from build123d import *

# Parameters (mm, degrees)
F2_W     = 2.54
F2_H     = 5.588
F3_DEPTH = 9.525
F5_D     = 3.2
F5_DEPTH = 7.5067


with BuildPart() as f1:
    # F0 (on Front) → F1 (revolve)
    with BuildSketch(Plane.XZ):
        Polygon((2.6, 17), (2.6, 0), (7.5057, 0), (7.5057, 15), (6.25, 15), (6.25, 17), align=None)
    revolve(axis=Axis((0, 0, 12.7238426358), (0, 0, -1)))

    # F2 (on face) → F3 (cut)
    with BuildSketch(Plane(origin=(0, 0, 0), x_dir=(1, 0, 0), z_dir=(0, 0, -1))):
        with Locations((5.08, 0)):
            Rectangle(F2_W, F2_H)
    extrude(amount=-F3_DEPTH, mode=Mode.SUBTRACT)

    # F5 (through all, one way)
    with BuildSketch(Plane(origin=(0, 0, 0), x_dir=(0, 1, 0), z_dir=(-1, 0, 0))):
        with Locations((0, -4.7625)):
            Circle(F5_D / 2)
    extrude(amount=-F5_DEPTH, mode=Mode.SUBTRACT)


solid = f1.part
CAD build for the part. Positions are in the model's coordinates, mm. A direction names the side the tool comes from. Round coordinates to 2 decimals unless told otherwise and drop trailing zeros. Write each loop counter-clockwise with the first axis right and the second up, starting at its lowest first coordinate (ties: lowest second). Pieces come first, ordered by that corner, then holes. Notation, with made-up numbers: (-4, 55.25) -> (43, 55.25) arc R22 ccw to (43, 67.25) -> close; hole circle Ø3 at (23.5, 21). An arc over 180 degrees is marked (long way). Answer as a JSON object with one key per item and string values.
(1) Pin check, flat tips, straight feed: P1, Ø3, axis at x = 5, z = 3.5, coming from the +Y side; P2, Ø3, axis at x = 5.5, z = 4.5, coming from the -Y side; P3, Ø1.5, axis at y = 3, z = 4.5, coming from the -X side. Stop position of each tip, or through.
Reported:
{"P1": "stops at y = 6.64", "P2": "stops at y = -6.35", "P3": "stops at x = -7.16"}
(2) Which spindle directions (+Z, -Z, +X, -X, +Y, -Y) get a long thin tool onto all of the face, cutting with end or side? Do faces 4 (the face through (-3, -6, 15)), 5 (the face through (6.35, 2, 5)), 6 (the face through (0, 3, 17)), 7 (the face through (-2.6, -0.1, 8.4)), 8 (the face through (3.11, -1.18, 3.68)). Say none if no direction does.
Reported:
{"face 4": "+Z", "face 5": "-Z", "face 6": "+Z, +X, -X, +Y, -Y", "face 7": "+Z, -Z", "face 8": "+X"}
(3) Band-saw the part on C-C, the plane y = -2.25. List the corners of the cut face in (x, z) (3 decimals).
Reported:
{"outline": "(-7.161, 0) -> (-1.303, 0) -> (-1.303, 17) -> (-5.831, 17) -> (-5.831, 15) -> (-7.161, 15) -> close; (1.303, 0) -> (3.81, 0) -> (3.81, 9.525) -> (6.35, 9.525) -> (6.35, 0) -> (7.161, 0) -> (7.161, 15) -> (5.831, 15) -> (5.831, 17) -> (1.303, 17) -> close"}
(4) Two-plate mould, pull along X, no slides. Class faces 1 (the face through (5, 2.794, 5)), 2 (the face through (5.96, -1.88, 16.01)), 3 (the face through (-3, 0, 0)): +X half, -X half, draft (parallel to the pull), parting line (faces both ways), or undercut.
Reported:
{"face 1": "undercut", "face 2": "parting line", "face 3": "draft"}
(5) Band-saw the part on B-B, the plane y = 0. Count the separate pieces of the cut face and the enclosed holes in it, then the cut area to 3 significant figures.
Reported:
{"separate pieces": "4", "enclosed holes": "0", "area": "130 mm^2"}
(6) Band-saw the part on A-A, the plane x = 0. List the corners of the cut face in (y, z), then the cut area to 3 significant figures.
Reported:
{"outline": "(-7.51, 0) -> (-2.6, 0) -> (-2.6, 17) -> (-6.25, 17) -> (-6.25, 15) -> (-7.51, 15) -> close; (2.6, 0) -> (7.51, 0) -> (7.51, 15) -> (6.25, 15) -> (6.25, 17) -> (2.6, 17) -> close", "area": "162 mm^2"}
(7) Probe probe 1 along X at (y, z) = (0, 12); probe 2 along Z at (x, y) = (3.1, 0); probe 3 along X at (y, z) = (-2, 8). List the from-to ranges inside material, lowest first. Write a range as [from, to].
Reported:
{"probe 1": "x = [-7.51, -2.6], [2.6, 7.51]", "probe 2": "z = [0, 3.16], [6.36, 17]", "probe 3": "x = [-7.23, -1.66], [1.66, 3.81], [6.35, 7.23]"}
(8) Band-saw the part on D-D, the plane z = 5. List the corners of the cut face in (x, y), then the cut area to 3 significant figures.
Reported:
{"outline": "(2.06, -1.58) arc R2.6 cw (long way) to (2.06, 1.58) -> (3.81, 1.58) -> (3.81, 2.79) -> (6.35, 2.79) -> (6.35, 1.58) -> (7.34, 1.58) arc R7.51 ccw (long way) to (7.34, -1.58) -> (6.35, -1.58) -> (6.35, -2.79) -> (3.81, -2.79) -> (3.81, -1.58) -> close", "area": "134 mm^2"}
